```python
from build123d import *

# Parameters (mm, degrees)
F3_R     = 5.665286
F3_R_2   = 7.253656
F3_R_3   = 6.669881
F4_DEPTH = 127
F6_R     = 7.910511
F6_R_2   = 7.431564
F6_R_3   = 6.884056
F7_DEPTH = 25.4


with BuildPart() as f1:
    # F0 (on Front) → F1 (revolve)
    with BuildSketch(Plane.XZ):
        with BuildLine():
            Line((-45.795509, 0), (-45.795509, -23.250027))
            Line((-45.795509, -23.250027), (-45.795509, -39.877315))
            Line((-45.795509, -39.877315), (0, -39.877315))
            Line((0, -39.877315), (0, -23.250027))
            Line((0, -23.250027), (0, 43.671444))
            ThreePointArc((0, 43.671444), (-29.841198, 41.661526), (-54.250058, 24.377299))
            Line((-54.250058, 24.377299), (-31.70458, 29.168213))
            Line((-31.70458, 29.168213), (-7.62, 30.238641))
            Line((-7.62, 30.238641), (-5.242722, -23.250027))
            Line((-5.242722, -23.250027), (-39.5955, -23.250027))
            Line((-39.5955, -23.250027), (-39.5955, 0))
            Line((-39.5955, 0), (-45.795509, 0))
        make_face()
    revolve(axis=Axis((0, 0, -2.677274), (0, 0, -1)))

    # F3 (on offset) → F4 (cut)
    with BuildSketch(Plane.XZ.offset(17.78)):
        with Locations((0, -19.800454)):
            Circle(F3_R)
        with Locations((20.878028, -11.179848)):
            Circle(F3_R_2)
        with Locations((-24.91894, -9.832879)):
            Circle(F3_R_3)
    extrude(amount=F4_DEPTH, mode=Mode.SUBTRACT)

    # F6 (on offset) → F7 (cut)
    with BuildSketch(Plane.YZ.offset(25.4)):
        with Locations((0, -21.147424)):
            Circle(F6_R)
        with Locations((-20.339243, -10.641061)):
            Circle(F6_R_2)
        with Locations((24.649547, -10.641061)):
            Circle(F6_R_3)
    extrude(amount=F7_DEPTH, mode=Mode.SUBTRACT)


solid = f1.part
```
Geometry: final body of the model. Coordinates: model frame, mm. A direction names the side the tool comes from. Give positions to 0.01 mm unless a question says otherwise; leave off trailing zeros. Loops run counter-clockwise (first coordinate to the right, second up) from the corner with the lowest first, then second, coordinate; pieces in that order, holes last. Notation, with made-up numbers: (83.25, -27.75) -> (140.25, -27.75) arc R8 cw to (140.25, -16.75) -> close; hole circle Ø5 at (42, -35). An arc over 180 degrees is marked (long way). Use one line per item in the form item = value.
Item 1: Section query A-A on x = -21. Give the number of separate pieces and of enclosed holes in the cut face, and give its area (3 significant figures).
A:
separate_pieces = 3
enclosed_holes = 0
area = 2,650 mm^2
Item 2: Access query for faces 1 (the face through (2.61, -37.82, -24.83)), 2 (the face through (35.971, -27.764, -10.314)), 3 (the face through (-37.77, 11.89, -11.46)). Directions: +Z, -Z, +X, -X, +Y, -Y. A direction counts if a zero-diameter tool reaches every point of the face in a straight line with its end or side. Return the directions, or none.
A:
face_1 = -Y
face_2 = +X
face_3 = none
Item 3: Pin query (flat end, axial travel): P1, Ø20.5, axis at y = 0, z = -21.15, coming from the -X side; P2, Ø9, axis at x = 0, z = -19.8, coming from the -Y side; P3, Ø5, axis at x = 20, z = -12.5, coming from the +Y side. Return the tip coordinate at first contact, or that it passes through.
A:
P1 = -45.8
P2 = -17.78
P3 = 42.32
Item 4: Section query B-B on z = 10. Output: boundary loops of the cut face in (x, y).
A:
outline = circle Ø13.44 at (0, 0)
Item 5: Line query: probe 1 along X at (y, z) = (1, -7); probe 2 along X at (y, z) = (0, -5.5); probe 3 along Z at (x, y) = (-4.5, -42). Output: solid intervals per line, ascending.
A:
probe_1 = -45.78 to -39.58, -5.88 to 5.88, 39.58 to 45.78
probe_2 = -45.8 to -39.6, -6.03 to 6.03, 39.6 to 45.8
probe_3 = -39.88 to -23.24, -16.36 to 0, 26.93 to 35.4
Item 6: Draft query along Z for faces 4 (the face through (-31.582, -32.811, -9.54)), 5 (the face through (1, 1, -39.877)). Return one class per face: pulls with the +Z half, pulls with the -Z half, needs draft (parallel to the pull), parting line crosses it, or undercut.
A:
face_4 = undercut
face_5 = pulls with the -Z half
